Could you check a few things on this model? Use its own coordinates, in mm. A direction names the side the tool comes from. Round coordinates to 2 decimals unless told otherwise and drop trailing zeros. Write each loop counter-clockwise with the first axis right and the second up, starting at its lowest first coordinate (ties: lowest second). Pieces come first, ordered by that corner, then holes. Notation, with made-up numbers: (62, 63.5) -> (91, 63.5) arc R16 ccw to (91, 81.5) -> close; hole circle Ø8 at (-38, 54.5). An arc over 180 degrees is marked (long way). Answer in a Markdown table with one row per item.
from build123d import *

# Parameters (mm, degrees)
SKETCH1_W            = 40.7
SKETCH1_H            = 20.2
BOSS_EXTRUDE1_DEPTH  = 34.5
BOSS_EXTRUDE2_DEPTH  = 2.6
FILLET2_R            = 1
FILLET2_OF_MIRROR1_R = 1
FILLET1_R            = 1
CHAMFER1_SIZE        = 1
SKETCH3_R            = 4
BOSS_EXTRUDE3_DEPTH  = 3


with BuildPart() as part:
    # Sketch1 → Boss-Extrude1 (new body)
    with BuildSketch(Plane.XY):
        Rectangle(SKETCH1_W, SKETCH1_H)
    extrude(amount=BOSS_EXTRUDE1_DEPTH)

    # Sketch2 → Boss-Extrude2 (add)
    with BuildSketch(Plane.XY.offset(5.5)):
        with BuildLine():
            Line((-20.35, 9), (-27.65, 9))
            Line((-27.65, 9), (-27.65, 6))
            Line((-27.65, 6), (-26.789553017, 6))
            ThreePointArc((-26.789553017, 6), (-22.95, 5), (-26.789553017, 4))
            Line((-26.789553017, 4), (-27.65, 4))
            Line((-27.65, 4), (-27.65, -4))
            Line((-27.65, -4), (-26.789553017, -4))
            ThreePointArc((-26.789553017, -4), (-22.95, -5), (-26.789553017, -6))
            Line((-26.789553017, -6), (-27.65, -6))
            Line((-27.65, -6), (-27.65, -9))
            Line((-27.65, -9), (-20.35, -9))
            Line((-20.35, -9), (-20.35, 9))
        make_face()
    boss_extrude2 = extrude(amount=-BOSS_EXTRUDE2_DEPTH)

    # Fillet2
    fillet2_edges = [part.edges().sort_by_distance(p)[0] for p in [
        (-27.65, -9, 4.2),
        (-27.65, 9, 4.2),
    ]]
    fillet(fillet2_edges, radius=FILLET2_R)

    # Mirror1: Boss-Extrude2 across plane
    add(boss_extrude2.mirror(Plane(origin=(0, 0, 0), x_dir=(0, 0, 1), z_dir=(1, 0, 0))))

    # Fillet2 of Mirror1
    fillet2_of_mirror1_edges = [part.edges().sort_by_distance(p)[0] for p in [
        (27.65, -9, 4.2),
        (27.65, 9, 4.2),
    ]]
    fillet(fillet2_of_mirror1_edges, radius=FILLET2_OF_MIRROR1_R)

    # Fillet1
    fillet1_edges = [part.edges().sort_by_distance(p)[0] for p in [
        (20.35, -10.1, 17.25),
        (-20.35, -10.1, 17.25),
        (-20.35, 10.1, 17.25),
        (20.35, 10.1, 17.25),
    ]]
    fillet(fillet1_edges, radius=FILLET1_R)

    # Chamfer1
    chamfer1_edges = [part.edges().sort_by_distance(p)[0] for p in [
        (-20.35, 0, 34.5),
        (20.35, 0, 34.5),
        (0, 10.1, 34.5),
        (-20.057106781, 9.807106781, 34.5),
        (20.057106781, 9.807106781, 34.5),
        (20.057106781, -9.807106781, 34.5),
        (-20.057106781, -9.807106781, 34.5),
        (0, -10.1, 34.5),
    ]]
    chamfer(chamfer1_edges, length=CHAMFER1_SIZE)

    # Sketch3 → Boss-Extrude3 (add)
    with BuildSketch(Plane(origin=(0, 0, 0), x_dir=(-1, 0, 0), z_dir=(0, 0, -1))):
        with Locations((10.35, 0)):
            Circle(SKETCH3_R)
    extrude(amount=BOSS_EXTRUDE3_DEPTH)


solid = part.part
1) Imagine slicing it at B-B, the plane z = 28. Please give me the cut outline in (x, y).
Findings:
| item | result |
|---|---|
| outline | (-20.35, -9.1) arc R1 ccw to (-19.35, -10.1) -> (19.35, -10.1) arc R1 ccw to (20.35, -9.1) -> (20.35, 9.1) arc R1 ccw to (19.35, 10.1) -> (-19.35, 10.1) arc R1 ccw to (-20.35, 9.1) -> close |
2) Imagine slicing it at C-C, the plane y = 5. Please give me the cut outline in (x, z).
Findings:
| item | result |
|---|---|
| outline | (-22.95, 2.9) -> (-20.35, 2.9) -> (-20.35, 0) -> (20.35, 0) -> (20.35, 2.9) -> (22.95, 2.9) -> (22.95, 5.5) -> (20.35, 5.5) -> (20.35, 33.5) -> (19.35, 34.5) -> (-19.35, 34.5) -> (-20.35, 33.5) -> (-20.35, 5.5) -> (-22.95, 5.5) -> close |
3) For faces 4 (the face through (-24, -9, 4)), 5 (the face through (24, 0, 5.5)), 6 (the face through (-24, 0, 5.5)), 7 (the face through (-14.045, -1.532, -1.479)), 8 (the face through (24, -9, 4)), which set-ups out of +Z, -Z, +X, -X, +Y, -Y let a thin tool reach every point of the face, with its end or its side?
Findings:
| item | result |
|---|---|
| face 4 | +Z, -Z, -X, -Y |
| face 5 | +Z, +X, +Y, -Y |
| face 6 | +Z, -X, +Y, -Y |
| face 7 | -Z |
| face 8 | +Z, -Z, +X, -Y |
4) Please list where these lines run through material, in increasing order: line 1 (Y direction, x = -25, z = 3.9); line 2 (Z direction, x = -5.5, y = 5.5); line 3 (X direction, y = -3.25, z = 13).
Findings:
| item | result |
|---|---|
| line 1 | y = -9 to -7.05, -2.95 to 2.95, 7.05 to 9 |
| line 2 | z = 0 to 34.5 |
| line 3 | x = -20.35 to 20.35 |
5) Imagine slicing it at A-A, the plane x = -25. Please give me the cut outline in (y, z), plus the area to 3 significant figures.
Findings:
| item | result |
|---|---|
| outline | (-9, 2.9) -> (-7.05, 2.9) -> (-7.05, 5.5) -> (-9, 5.5) -> close; (-2.95, 2.9) -> (2.95, 2.9) -> (2.95, 5.5) -> (-2.95, 5.5) -> close; (7.05, 2.9) -> (9, 2.9) -> (9, 5.5) -> (7.05, 5.5) -> close |
| area | 25.5 mm^2 |
6) Imagine slicing it at D-D, the plane x = -10.35. Please give me the cut outline in (y, z).
Findings:
| item | result |
|---|---|
| outline | (-10.1, 0) -> (-4, 0) -> (-4, -3) -> (4, -3) -> (4, 0) -> (10.1, 0) -> (10.1, 33.5) -> (9.1, 34.5) -> (-9.1, 34.5) -> (-10.1, 33.5) -> close |
7) For pin 1 (5.5 mm diameter, centred on y = 4.5, z = 22, fed in from +X); pin 2 (4 mm diameter, centred on x = 3, y = 1.5, fed in from -Z); pin 3 (4.5 mm diameter, centred on x = 25, y = 5, fed in from -Z), each with a flat end and sliding along its axis, tell me the tip position at first contact or that it passes through.
Findings:
| item | result |
|---|---|
| pin 1 | stops at x = 20.35 |
| pin 2 | stops at z = 0 |
| pin 3 | stops at z = 2.9 |
8) Thinking about a two-plate mould opening in Y: for faces 1 (the face through (-22.95, 5.08, 4.22)), 2 (the face through (23, 9, 4)), 3 (the face through (0, 0, 0)), which applies, +Y half, -Y half, draft (parallel to the pull), parting line (faces both ways), or undercut?
Findings:
| item | result |
|---|---|
| face 1 | undercut |
| face 2 | +Y half |
| face 3 | draft |
